The model under review builds one solid part; all positions refer to its coordinate system, in mm. Face numbers are marked on the shaded views. A direction names the side the tool comes from. Coordinates: 2 decimals unless noted, no trailing zeros. Write each loop counter-clockwise with the first axis right and the second up, starting at its lowest first coordinate (ties: lowest second). Pieces come first, ordered by that corner, then holes. Notation, with made-up numbers: (19.5, -29.5) -> (38.5, -29.5) arc R25 cw to (38.5, -2.5) -> close; hole circle Ø8 at (-16.5, 84). An arc over 180 degrees is marked (long way). Write each question's results on one line, items separated by ' | '.
```python
from build123d import *

# Parameters (mm, degrees)
F1_DEPTH = 63.5
F0_W     = 35.7702043533
F0_H     = 19.0499988828
F2_DEPTH = 25.4
F3_DEPTH = 7.9375
F5_R     = 6.35


# Not quite as in the source:
# - ends of sketch curves that miss each other by under 0.0002 mm in the source are joined


with BuildPart() as f1:
    # F0 (on Front) → F1 (new body, symmetric)
    with BuildSketch(Plane.XZ):
        Polygon((-41.275, -9.525), (41.275, -9.525), (41.275, 9.525), (22.225, 9.525), (-41.275, 9.525), align=None)
    extrude(amount=F1_DEPTH, both=True)

    # F0 (on Front) → F2 (join, symmetric)
    with BuildSketch(Plane.XZ):
        with BuildLine():
            Line((22.225, 9.525), (41.275, 9.525))
            Line((41.275, 9.525), (41.275, 27.0002))
            ThreePointArc((41.275, 27.0002), (45.9246798487, 38.2255201513), (57.15, 42.8752))
            Line((57.15, 42.8752), (60.325, 42.8752))
            Line((60.325, 42.8752), (60.325, 61.9251988828))
            Line((60.325, 61.9251988828), (57.15, 61.9251988828))
            add(Edge.make_bspline(
                [(55.0732880095, 61.8634025538), (55.7666834516, 61.8883145564), (56.4589847756, 61.9089220973), (57.15, 61.9251988828)],
                knots=[109.8121329902, 109.8121329902, 109.8121329902, 109.8121329902, 111.5045361635, 111.5045361635, 111.5045361635, 111.5045361635], degree=3))
            ThreePointArc((55.0732880095, 61.8634025538), (31.7306688594, 50.9504239941), (22.225, 27.0002))
            Line((22.225, 27.0002), (22.225, 9.525))
        make_face()
        with Locations((78.2101021767, 52.4001994414)):
            Rectangle(F0_W, F0_H)
    extrude(amount=F2_DEPTH, both=True)

    # F0 (on Front) → F3 (join, symmetric)
    with BuildSketch(Plane.XZ):
        with BuildLine():
            add(Edge.make_bspline(
                [(-41.275, 9.525), (-39.5154446815, 40.5083175564), (10.0820981423, 60.2469791277), (55.0732880095, 61.8634025538)],
                knots=[0, 0, 0, 0, 109.8121329902, 109.8121329902, 109.8121329902, 109.8121329902], degree=3))
            Line((-41.275, 9.525), (22.225, 9.525))
            Line((22.225, 9.525), (22.225, 27.0002))
            ThreePointArc((22.225, 27.0002), (31.7306688594, 50.9504239941), (55.0732880095, 61.8634025538))
        make_face()
    extrude(amount=F3_DEPTH, both=True)

    # F0 (on Front) → F4 (revolve)
    with BuildSketch(Plane.XZ):
        Polygon((96.0952043533, 61.9251988828), (96.0952043533, 42.8752), (96.0952043533, 38.1), (111.125, 38.1), (111.125, 66.675), (96.0952043533, 66.675), align=None)
    revolve(axis=Axis((96.0952043533, 0, 52.3875), (0, 0, -1)))

    # F5
    f5_edges = [f1.edges().sort_by_distance(p)[0] for p in [
        (41.275, -63.5, 0),
        (-41.275, -63.5, 0),
        (41.275, 63.5, 0),
        (-41.275, 63.5, 0),
    ]]
    fillet(f5_edges, radius=F5_R)


solid = f1.part
```
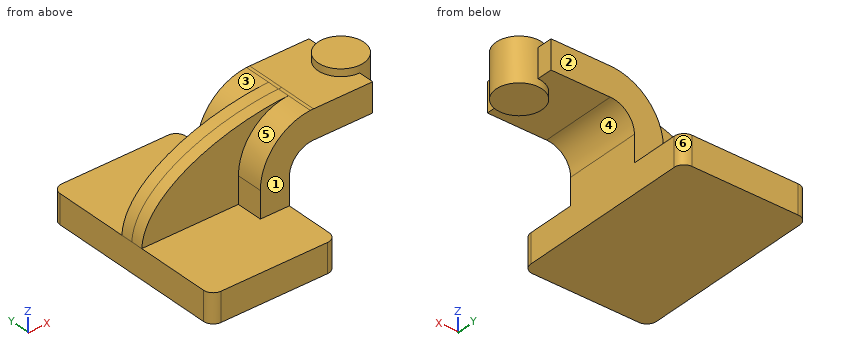
Q1. Clearance check with flat-ended pins moving along their axes: P1, Ø15, axis at x = 92.5, y = -1.5, coming from the -Z side; P2, Ø8.5, axis at y = -19, z = 19, coming from the -X side (3 decimals); P3, Ø8.5, axis at y = 20.5, z = 54, coming from the +X side; P4, Ø2, axis at y = -26.5, z = 28, coming from the -X side. State where each tip first meets the part, or that it passes through.
Solution:
P1: z = 38.1 | P2: x = 22.225 | P3: x = 96.1 | P4: through
Q2. Add section A-A (y = 44.5). Write out the cut boundary in (x, z) (3 decimals), plus the area to 3 significant figures.
Solution:
outline: (-41.275, -9.525) -> (41.275, -9.525) -> (41.275, 9.525) -> (-41.275, 9.525) -> close | area: 1,570 mm²
Q3. Add section B-B (x = 98.5). Write out the cut boundary in (y, z) (3 decimals), plus the area to 3 significant figures.
Solution:
outline: (-14.836, 38.1) -> (14.836, 38.1) -> (14.836, 66.675) -> (-14.836, 66.675) -> close | area: 848 mm²
Q4. For line 1 (Z direction, x = 94, y = -8) (3 decimals); line 2 (Y direction, x = -30.5, z = 28); line 3 (Z direction, x = 21, y = 9) (3 decimals), list the stretches that pass through material, from the lowest coordinate up. Write a range as from..to.
Solution:
line 1: 38.1..66.675 | line 2: -7.94..7.94 | line 3: -9.525..9.525
Q5. Machinability: for the marked faces 1, 2 and 3, which of the approach directions +Z, -Z, +X, -X, +Y, -Y give a long, thin tool a straight path to every point of the face, cutting with its end or side? Answer none if there is none.
Solution:
face 1: +Z, +X, -X, -Y | face 2: +Z, +X, -X, +Y | face 3: +Z, -X, +Y
Q6. Draft analysis for pull direction X (two halves, no side actions). For the marked faces 4, 5 and 6, state which applies: pulls with the +X half, pulls with the -X half, needs draft (parallel to the pull), parting line crosses it, or undercut.
Solution:
face 4: undercut | face 5: pulls with the -X half | face 6: pulls with the +X half
